from build123d import *

# Parameters (mm, degrees)
SKETCH1_R               = 28.575
SKETCH1_R_2             = 2.286
SKETCH1_R_3             = 1.5875
SKETCH1_R_4             = 1.143
SKETCH1_R_5             = 1.397
SKETCH1_R_6             = 2.159
BOSS_EXTRUDE1_DEPTH     = 6.35
SKETCH2_R               = 4.191
SKETCH2_R_2             = 3.81
CUT_EXTRUDE1_DEPTH      = 3.175
SKETCH3_R               = 3.6576
CUT_EXTRUDE2_DEPTH      = 4.572
CHAMFER1_SIZE           = 0.3175
CUT_EXTRUDE_THIN2_DEPTH = 0.254
FILLET1_R               = 0.3175
CUT_EXTRUDE_THIN1_DEPTH = 0.254
CHAMFER2_SIZE           = 0.635


# Some blends are built 0.0001 mm under size
with BuildPart() as part:
    # Sketch1 → Boss-Extrude1 (new body)
    with BuildSketch(Plane.XY):
        Circle(SKETCH1_R)
        with Locations((0, 19.05)):
            Circle(SKETCH1_R_2, mode=Mode.SUBTRACT)
        with Locations((14.893889741, 11.877480725)):
            Circle(SKETCH1_R_3, mode=Mode.SUBTRACT)
        with Locations((18.572376727, -4.239023792)):
            Circle(SKETCH1_R_4, mode=Mode.SUBTRACT)
        with Locations((8.26548523, -17.163456934)):
            Circle(SKETCH1_R_3, mode=Mode.SUBTRACT)
        with Locations((-8.26548523, -17.163456934)):
            Circle(SKETCH1_R_5, mode=Mode.SUBTRACT)
        with Locations((-18.572376727, -4.239023792)):
            Circle(SKETCH1_R_4, mode=Mode.SUBTRACT)
        with Locations((-14.893889741, 11.877480725)):
            Circle(SKETCH1_R_4, mode=Mode.SUBTRACT)
        Circle(SKETCH1_R_6, mode=Mode.SUBTRACT)
    extrude(amount=BOSS_EXTRUDE1_DEPTH)

    # Sketch2 → Cut-Extrude1 (cut)
    with BuildSketch(Plane.XY.offset(6.35)):
        with Locations((0, 19.05)):
            Circle(SKETCH2_R)
        with Locations((14.893889741, 11.877480725)):
            Circle(SKETCH2_R_2)
        with Locations((18.572376727, -4.239023792)):
            Circle(SKETCH2_R_2)
        with Locations((8.26548523, -17.163456934)):
            Circle(SKETCH2_R)
        with Locations((-8.26548523, -17.163456934)):
            Circle(SKETCH2_R_2)
        with Locations((-18.572376727, -4.239023792)):
            Circle(SKETCH2_R_2)
        with Locations((-14.893889741, 11.877480725)):
            Circle(SKETCH2_R_2)
    extrude(amount=-CUT_EXTRUDE1_DEPTH, mode=Mode.SUBTRACT)

    # Sketch3 → Cut-Extrude2 (cut)
    with BuildSketch(Plane.XY.offset(6.35)):
        Circle(SKETCH3_R)
    extrude(amount=-CUT_EXTRUDE2_DEPTH, mode=Mode.SUBTRACT)

    # Chamfer1
    chamfer1_edges = [part.edges().sort_by_distance(p)[0] for p in [
        (17.429376727, -4.239023792, 0),
        (6.67798523, -17.163456934, 0),
        (-28.575, 0, 0),
        (-9.66248523, -17.163456934, 0),
        (-19.715376727, -4.239023792, 0),
        (-16.036889741, 11.877480725, 0),
        (-2.159, 0, 0),
        (-28.575, 0, 6.35),
        (11.083889741, 11.877480725, 3.175),
        (13.306389741, 11.877480725, 3.175),
        (11.083889741, 11.877480725, 6.35),
        (13.306389741, 11.877480725, 0),
        (14.762376727, -4.239023792, 3.175),
        (17.429376727, -4.239023792, 3.175),
        (14.762376727, -4.239023792, 6.35),
        (4.07448523, -17.163456934, 3.175),
        (6.67798523, -17.163456934, 3.175),
        (4.07448523, -17.163456934, 6.35),
        (-12.07548523, -17.163456934, 3.175),
        (-9.66248523, -17.163456934, 3.175),
        (-12.07548523, -17.163456934, 6.35),
        (-22.382376727, -4.239023792, 3.175),
        (-19.715376727, -4.239023792, 3.175),
        (-22.382376727, -4.239023792, 6.35),
        (-18.703889741, 11.877480725, 3.175),
        (-16.036889741, 11.877480725, 3.175),
        (-18.703889741, 11.877480725, 6.35),
        (-4.191, 19.05, 3.175),
        (-2.286, 19.05, 3.175),
        (-4.191, 19.05, 6.35),
        (-2.159, 0, 1.778),
        (-3.6576, 0, 6.35),
        (-2.286, 19.05, 0),
    ]]
    chamfer(chamfer1_edges, length=CHAMFER1_SIZE)

    # Sketch5 → Cut-Extrude-Thin2 (cut)
    with BuildSketch(Plane.XY.offset(6.35)):
        Polygon((5.103012367, 3.663418823), (10.06764228, 7.622579065), (9.671726256, 8.119042056), (4.707096343, 4.159881815), align=None)
        Polygon((9.615180928, 3.606873495), (5.656020686, 8.571503409), (5.159557695, 8.175587385), (9.118717937, 3.210957471), align=None)
        Polygon((-9.615180928, -3.606873495), (-5.656020686, -8.571503409), (-5.159557695, -8.175587385), (-9.118717937, -3.210957471), align=None)
    extrude(amount=-CUT_EXTRUDE_THIN2_DEPTH, mode=Mode.SUBTRACT)

    # Fillet1
    fillet1_edges = [part.edges().sort_by_distance(p)[0] for p in [
        (-5.656020686, -8.571503409, 6.223),
        (-9.615180928, -3.606873495, 6.223),
        (-9.118717937, -3.210957471, 6.223),
        (-5.159557695, -8.175587385, 6.223),
        (10.06764228, 7.622579065, 6.223),
        (9.615180928, 3.606873495, 6.223),
        (9.118717937, 3.210957471, 6.223),
        (5.103012367, 3.663418823, 6.223),
        (4.707096343, 4.159881815, 6.223),
        (5.159557695, 8.175587385, 6.223),
        (9.671726256, 8.119042056, 6.223),
        (5.656020686, 8.571503409, 6.223),
        (7.337095828, 5.445040932, 6.223),
        (7.833558819, 5.840956956, 6.223),
        (7.437642795, 6.337419948, 6.223),
        (6.941179804, 5.941503923, 6.223),
    ]]
    fillet(fillet1_edges, radius=FILLET1_R - 0.0001)  # a hair under: the kernel refuses the full size

    # Sketch4 → Cut-Extrude-Thin1 (cut)
    with BuildSketch(Plane.XY.offset(6.35)):
        Polygon((-13.113371884, 25.400790182), (-0.636538078, -0.507622178), (21.845939581, -18.436799827), (22.835729642, -17.195642349), (0.636538078, 0.507622178), (-11.683083806, 26.089580618), align=None)
    extrude(amount=-CUT_EXTRUDE_THIN1_DEPTH, mode=Mode.SUBTRACT)

    # Chamfer2
    # the kernel refuses this chamfer: 0.635 mm, written as the material it takes off along each edge
    with BuildSketch(Plane(origin=(1.273628889, -2.030929502, 6.35), x_dir=(-0.6232540709086805, -0.7815358852062859, 0.027495876610585914), z_dir=(0.7818314824680229, -0.6234898018587423, 0))) as chamfer2_piece_1_section:
        Polygon((CHAMFER2_SIZE * 0.999621916911, CHAMFER2_SIZE * 0.0274958766106), (-CHAMFER2_SIZE * 0.0274958766106, CHAMFER2_SIZE * 0.999621916911), (0, 0), align=None)
    chamfer2_piece_1 = extrude(amount=27.617341328, mode=Mode.PRIVATE)
    chamfer2_piece_1 = split(chamfer2_piece_1, bisect_by=Plane(origin=(11.905816468, -10.845976149, 6.096), z_dir=(0, 0, 1)), keep=Keep.TOP, mode=Mode.PRIVATE)
    add(chamfer2_piece_1, mode=Mode.SUBTRACT)
    with BuildSketch(Plane(origin=(23.855525862, -18.008902696, 6.35), x_dir=(0.6232540709086805, 0.7815358852062859, 0.027495876610585834), z_dir=(-0.7818314824680228, 0.6234898018587423, 0))) as chamfer2_piece_2_section:
        Polygon((CHAMFER2_SIZE * 0.999621916911, CHAMFER2_SIZE * 0.0274958766106), (-CHAMFER2_SIZE * 0.0274958766106, CHAMFER2_SIZE * 0.999621916911), (0, 0), align=None)
    chamfer2_piece_2 = extrude(amount=27.617341328, mode=Mode.PRIVATE)
    chamfer2_piece_2 = split(chamfer2_piece_2, bisect_by=Plane(origin=(13.223338283, -9.193856049, 6.096), z_dir=(0, 0, 1)), keep=Keep.TOP, mode=Mode.PRIVATE)
    add(chamfer2_piece_2, mode=Mode.SUBTRACT)
    with BuildSketch(Plane(origin=(-0.266312692, 2.382411119, 6.35), x_dir=(0.9006282268100128, 0.4337196950133434, 0.02749587661058592), z_dir=(-0.43388373911756706, 0.9009688679024148, 0))) as chamfer2_piece_3_section:
        Polygon((CHAMFER2_SIZE * 0.999621916911, CHAMFER2_SIZE * 0.0274958766106), (-CHAMFER2_SIZE * 0.0274958766106, CHAMFER2_SIZE * 0.999621916911), (0, 0), align=None)
    chamfer2_piece_3 = extrude(amount=27.617341328, mode=Mode.PRIVATE)
    chamfer2_piece_3 = split(chamfer2_piece_3, bisect_by=Plane(origin=(-6.020877298, 14.937627019, 6.096), z_dir=(0, 0, 1)), keep=Keep.TOP, mode=Mode.PRIVATE)
    add(chamfer2_piece_3, mode=Mode.SUBTRACT)
    with BuildSketch(Plane(origin=(-13.679316089, 26.575985434, 6.35), x_dir=(0.024772928821820563, 0.01193001375411458, -0.999621916911297), z_dir=(0.43388373911756706, -0.9009688679024149, 0))) as chamfer2_piece_4_section:
        Polygon((CHAMFER2_SIZE * 0.999621916911, -CHAMFER2_SIZE * 0.0274958766106), (-CHAMFER2_SIZE * 0.0274958766106, -CHAMFER2_SIZE * 0.999621916911), (0, 0), align=None)
    chamfer2_piece_4 = extrude(amount=27.617341328, mode=Mode.PRIVATE)
    chamfer2_piece_4 = split(chamfer2_piece_4, bisect_by=Plane(origin=(-7.924751483, 14.020769534, 6.096), z_dir=(0, 0, 1)), keep=Keep.TOP, mode=Mode.PRIVATE)
    add(chamfer2_piece_4, mode=Mode.SUBTRACT)


solid = part.part
Here's how the part is built. I have some questions about the finished solid (model axes, mm). A direction names the side the tool comes from. Coordinates: 2 decimals unless noted, no trailing zeros.
1. For P1, Ø4, axis at x = -2, y = 20.5, coming from the +Z side; P2, Ø1.5, axis at y = 5, z = 4, coming from the +X side; P3, Ø6.5, axis at x = 8.27, y = -17.16, coming from the +Z side (3 decimals), each with a flat end and sliding along its axis, tell me the tip position at first contact or that it passes through.
2. For faces 1 (the cylindrical face through (17.43, -4.19, 1.57)), 2 (the flat face through (-15, 10, 3.175)), which set-ups out of +Z, -Z, +X, -X, +Y, -Y let a thin tool reach every point of the face, with its end or its side?
3. If we mould it in two halves opening along X, with no side actions, what happens to faces 3 (the flat face through (8, 11, 6.35)), 4 (the flat face through (-9, -19, 3.175))? For each: pulls with the +X half, pulls with the -X half, needs draft (parallel to the pull), parting line crosses it, or undercut.
4. I need wall thicknesses on L1, parallel to Y at x = -3, z = 4.5; L2, parallel to X at y = -15, z = 4; L3, parallel to X at y = 16.5, z = 4.5. Which ranges of each line are inside material? Lowest first, please.
Taken from the geometry:
1. P1: stops at z = 6.31
1. P2: stops at x = 28.26
1. P3: stops at z = 3.175
2. face 1: +Z, -Z
2. face 2: +Z
3. face 3: needs draft
3. face 4: undercut
4. L1: y = -28.42 to -2.09, 2.09 to 16.12, 21.98 to 28.42
4. L2: x = -24.32 to -11.4, -5.13 to 4.68, 11.85 to 24.32
4. L3: x = -23.33 to -3.33, 3.33 to 23.33
